Geometry check sheet. Reference: the model listing, model coordinates, mm. A direction names the side the tool comes from. Give positions to 0.01 mm unless a question says otherwise; leave off trailing zeros. Loops run counter-clockwise (first coordinate to the right, second up) from the corner with the lowest first, then second, coordinate; pieces in that order, holes last.
1. Cross-section at B-B, the plane x = 0.25. Record the cut outline in (y, z).
2. Release check for a two-part mould opening along Y. For faces 1 (the flat face through (0.616, -1.088, -0.986)), 2 (the cylindrical face through (-3.233, -1.341, -1.972)), 3 (the flat face through (0, 0, -9)) record: +Y half, -Y half, draft (parallel to the pull), parting line (faces both ways), or undercut.
3. Cross-section at C-C, the plane z = -7.25. Record the cut outline in (x, y), plus the area to 3 significant figures.
4. Cross-section at A-A, the plane y = 0. Record the cut outline in (x, z), plus the area to 3 significant figures.
5. Cross-section at D-D, the plane y = -1.75. Record the cut outline in (x, z), plus the area to 3 significant figures.
6. Go/stop test with flat-tipped pins: pin 1 Ø1 at (y, z) = (0.5, -6) entering from -X; pin 2 Ø2 at (x, y) = (0.5, -0.5) entering from +Z; pin 3 Ø4 at (x, z) = (0.5, -7.5) entering from -Y. Record where each tip stops, or that it passes through.
7. Tool access check on faces 4 (the flat face through (1.25, 0, -1)), 5 (the flat face through (0, -2, 0)), 6 (the flat face through (-2, -2, -4)). Record the directions out of +Z, -Z, +X, -X, +Y, -Y that give a thin tool (end or side, any length) a straight path to the whole face; none if there is none.
8. Material ranges on L1, parallel to Z at x = -0.5, y = 2; L2, parallel to Z at x = 1, y = 0.25; L3, parallel to X at y = -0.75, z = -0.5, recorded low to high.
from build123d import *

# Parameters (mm, degrees)
CYLINDER028_R                      = 2
CYLINDER028_DEPTH                  = 9
CYLINDER027_R                      = 3.5
CYLINDER027_DEPTH                  = 4
FUSION001018017024_PLACEMENT_ANGLE = 180
POCKET002018004005005017010_DEPTH  = 2


with BuildPart() as cylinder028:
    # Cylinder028 → Cylinder028 (new body)
    with BuildSketch(Plane.XY):
        Circle(CYLINDER028_R)
    extrude(amount=CYLINDER028_DEPTH)


with BuildPart() as zylinderkopfschraube_m4x6_din912:
    # Cylinder027 → Cylinder027 (new body)
    with BuildSketch(Plane.XY):
        Circle(CYLINDER027_R)
    extrude(amount=CYLINDER027_DEPTH)

    # Fusion001018017024: union Cylinder028
    add(cylinder028.part)


with BuildPart() as zylinderkopfschraube_m4x6_din912_1:
    # Fusion001018017024 placement: moved
    add(zylinderkopfschraube_m4x6_din912.part.rotate(Axis((0, 0, 0), (0, 1, 0)), FUSION001018017024_PLACEMENT_ANGLE))

    # Sketch028 → Pocket002018004005005017010 (cut)
    with BuildSketch(Plane(origin=(0, 0, 0), x_dir=(-1, 0, 0), z_dir=(0, 0, 1))):
        Polygon((1.25, -0.721688), (1.25, 0.721688), (0, 1.443376), (-1.25, 0.721688), (-1.25, -0.721688), (0, -1.443376), align=None)
    extrude(amount=-POCKET002018004005005017010_DEPTH, mode=Mode.SUBTRACT)


solid = zylinderkopfschraube_m4x6_din912_1.part
Result:
1. outline: (-3.49, -4) - (-1.98, -4) - (-1.98, -9) - (1.98, -9) - (1.98, -4) - (3.49, -4) - (3.49, 0) - (1.3, 0) - (1.3, -2) - (-1.3, -2) - (-1.3, 0) - (-3.49, 0) - close
2. face 1: undercut
2. face 2: parting line
2. face 3: draft
3. outline: circle Ø4 at (0, 0)
3. area: 12.6 mm2
4. outline: (-3.5, -4) - (-2, -4) - (-2, -9) - (2, -9) - (2, -4) - (3.5, -4) - (3.5, 0) - (1.25, 0) - (1.25, -2) - (-1.25, -2) - (-1.25, 0) - (-3.5, 0) - close
4. area: 43.0 mm2
5. outline: (-3.03, -4) - (-0.97, -4) - (-0.97, -9) - (0.97, -9) - (0.97, -4) - (3.03, -4) - (3.03, 0) - (-3.03, 0) - close
5. area: 33.9 mm2
6. pin 1: stops at x = -2
6. pin 2: stops at z = 0
6. pin 3: stops at y = -2
7. face 4: +Z
7. face 5: +Z, +X, -X, +Y, -Y
7. face 6: -Z
8. L1: z = -4 to 0
8. L2: z = -9 to -2
8. L3: x = -3.42 to -1.2, 1.2 to 3.42
